from build123d import *

# Parameters (mm, degrees)
F1_DEPTH = 5
F2_D     = 3.3
F3_R     = 5


with BuildPart() as f1:
    # F0 (on Top) → F1 (new body)
    with BuildSketch(Plane.XY):
        Polygon((115.4999993443, 64.5), (103, 64.5), (-101, 64.5), (-101, -63.5), (103, -63.5), (115.4999993443, -63.5), (115.4999993443, -43.5), (106.9999993443, -43.5), (106.9999993443, -55), (103, -55), (-92.5, -55), (-92.5, 56), (103, 56), (106.9999993443, 56), (106.9999993443, 39.5), (115.4999993443, 39.5), align=None)
    extrude(amount=F1_DEPTH)

    # F2 (through all)
    with Locations(Plane(origin=(0, 0, 0), x_dir=(1, 0, 0), z_dir=(0, 0, -1))):
        with Locations((-97, -60.5), (99, -60.5), (99, 59.5), (-97, 59.5)):
            Hole(F2_D / 2)

    # F3
    f3_edges = [f1.edges().sort_by_distance(p)[0] for p in [
        (115.499999, 39.5, 2.5),
        (115.499999, 64.5, 2.5),
        (-101, 64.5, 2.5),
        (-101, -63.5, 2.5),
        (115.499999, -63.5, 2.5),
        (115.499999, -43.5, 2.5),
    ]]
    fillet(f3_edges, radius=F3_R)


solid = f1.part
Build history of the part. All positions in model axes, mm. A direction names the side the tool comes from. Round coordinates to 2 decimals unless told otherwise and drop trailing zeros. Order: outer loops, then holes, each group sorted by start corner. A loop starts at its lowest first (then second) coordinate and runs counter-clockwise, first axis right, second up. Notation, with made-up numbers: M 79.25,-31 L 137.25,-31 A18 cw 137.25,-17 Z; hole C 78.5,81.25 d6. An arc over 180 degrees is marked long. Use CSV: the item, a comma, the result in double quotes. Start each with the question number.
(1) Cut at A-A on x = 62. List the corners of the cut face in (y, z).
(2) Flat gauge pin, fed straight in: P1, Ø3, axis at y = -12, z = 4, coming from the +X side. Where does the tip first touch, or does it go through?
(3) Tool access for faces 4 (the face through (107, -49, 2)), 5 (the face through (-1, 58, 0)), 6 (the face through (114.07, 41, 2.54)): list every direction of +Z, -Z, +X, -X, +Y, -Y with a clear straight run to the whole face (end or side of a thin tool).
(4) Cut at C-C on z = 1.05. List the corners of the cut face in (x, y).
(5) Cut at B-B on y = 51.5. List the corners of the cut face in (x, z).
(6) Drill centre lines: probe 1 along Y at (x, z) = (99, 1.35); probe 2 along Y at (x, z) = (-22, 2.05); probe 3 along X at (y, z) = (-59.5, 2.5). Where is each one in solid material? Low to high.
(7) Mould opens along X. For faces 1 (the face through (-101, 1, 2)), 2 (the face through (107, 48, 2)), 3 (the face through (6, -63.5, 2)) say: +X half, -X half, draft (parallel to the pull), parting line (faces both ways), or undercut.
(8) Cut at D-D on y = -41. List the corners of the cut face in (x, z), then the cut area to 3 significant figures.
Findings:
1,outline,"M -63.5,0 L -55,0 L -55,5 L -63.5,5 Z; M 56,0 L 64.5,0 L 64.5,5 L 56,5 Z"
2,P1,"stops at x = -92.5"
3,face 4,"+Z, -Z"
3,face 5,"-Z, +X, -X, +Y, -Y"
3,face 6,"+Z, -Z, +X"
4,outline,"M -101,-58.5 A5 ccw -96,-63.5 L 110.5,-63.5 A5 ccw 115.5,-58.5 L 115.5,-48.5 A5 ccw 110.5,-43.5 L 107,-43.5 L 107,-55 L -92.5,-55 L -92.5,56 L 107,56 L 107,39.5 L 110.5,39.5 A5 ccw 115.5,44.5 L 115.5,59.5 A5 ccw 110.5,64.5 L -96,64.5 A5 ccw -101,59.5 Z; hole C -97,-59.5 d3.3; hole C -97,60.5 d3.3; hole C 99,-59.5 d3.3; hole C 99,60.5 d3.3"
5,outline,"M -101,0 L -92.5,0 L -92.5,5 L -101,5 Z; M 107,0 L 115.5,0 L 115.5,5 L 107,5 Z"
6,probe 1,"y = -63.5 to -61.15, -57.85 to -55, 56 to 58.85, 62.15 to 64.5"
6,probe 2,"y = -63.5 to -55, 56 to 64.5"
6,probe 3,"x = -100.9 to -98.65, -95.35 to 97.35, 100.65 to 115.4"
7,face 1,"-X half"
7,face 2,"undercut"
7,face 3,"draft"
8,outline,"M -101,0 L -92.5,0 L -92.5,5 L -101,5 Z"
8,area,"42.5 mm^2"
